Build history of the part. All positions in model axes, mm. Give positions to 0.01 mm unless a question says otherwise; leave off trailing zeros. Write each loop counter-clockwise with the first axis right and the second up, starting at its lowest first coordinate (ties: lowest second). Pieces come first, ordered by that corner, then holes. Notation, with made-up numbers: (60, 45) -> (70, 45) arc R28 ccw to (70, 70) -> close; hole circle Ø9 at (12.25, 36.25). An arc over 180 degrees is marked (long way). Write item = value, one per line. Start each with the question number.
Q1. Wall check: line 1 (Y direction, x = 50.8, z = 83.95); line 2 (X direction, y = 101.5, z = 83.9); line 3 (Y direction, x = 75.5, z = 84.2). Give the ranges that are in metal, low to high.
Q2. Mould opens along X. For faces 1 (the face through (88, 116, 85.725)), 2 (the face through (50.068, 198.315, 84.115)) say: pulls with the +X half, pulls with the -X half, needs draft (parallel to the pull), parting line crosses it, or undercut.
Q3. Drop a flat-ended pin along its axis: P1, Ø4, axis at x = 26.99, y = 127, coming from the -Z side (3 decimals). Give the stop position or say it passes through.
Q4. Saw through at B-B, the plane y = 177.8. List the corners of the cut face in (x, z) (3 decimals).
Q5. Saw through at A-A, the plane x = 127. List the corners of the cut face in (y, z) (3 decimals), then the cut area to 3 significant figures.
from build123d import *

# Parameters (mm, degrees)
F0_W      = 50.8
F0_H      = 177.8
F1_DEPTH  = 3.175
F3_DEPTH  = 76.2
F5_DEPTH  = 3.175
F7_D      = 6.7564
F7_DEPTH  = 29.21
F7_TIP    = 2.0298273432
F8_W      = 127
F8_H      = 177.8
F8_R      = 3.3782
F9_DEPTH  = 3.175
F10_W     = 247.0957003534
F10_H     = 423.9609837532
F11_DEPTH = 82.55


# Not quite as in the source:
# - an extrude ends at something that could not be found from the text; its depth is read off the source's solid


with BuildPart() as f1:
    # F0 (on Top) → F1 (new body)
    with BuildSketch(Plane.XY):
        Polygon((0, 228.6), (0, 177.8), (50.8, 177.8), (177.8, 177.8), (177.8, 228.6), align=None)
        with Locations((25.4, 88.9)):
            Rectangle(F0_W, F0_H)
    extrude(amount=F1_DEPTH)

    # F2 (on face) → F3 (join)
    with BuildSketch(Plane.XY.offset(3.175)):
        Polygon((3.175, 0), (3.175, 225.425), (177.8, 225.425), (177.8, 228.6), (0, 228.6), (0, 0), align=None)
    extrude(amount=F3_DEPTH)

    # F4 (on face) → F5 (join)
    with BuildSketch(Plane.XY.offset(79.375)):
        Polygon((177.8, 228.6), (0, 228.6), (0, 0), (3.175, 0), (3.175, 225.425), (177.8, 225.425), align=None)
        Polygon((177.8, 177.8), (177.8, 225.425), (3.175, 225.425), (3.175, 0), (50.8, 0), (50.8, 177.8), align=None)
    extrude(amount=F5_DEPTH)

    # F7
    with Locations(Plane.XY.offset(82.55)):
        with Locations((26.9875, 25.4), (26.9875, 50.8), (26.9875, 76.2), (26.9875, 101.6), (26.9875, 127), (26.9875, 152.4), (26.9875, 177.8), (50.8, 201.6125), (76.2, 201.6125), (101.6, 201.6125), (127, 201.6125), (152.4, 201.6125)):
            Hole(F7_D / 2, depth=F7_DEPTH)
            with Locations((0, 0, -(F7_DEPTH + F7_TIP / 2))):  # 118° drill point
                Cone(0, F7_D / 2, F7_TIP, mode=Mode.SUBTRACT)

    # F8 (on face) → F9 (join)
    with BuildSketch(Plane.XY.offset(82.55)):
        with Locations((114.3, 88.9)):
            Rectangle(F8_W, F8_H)
        Polygon((0, 228.6), (0, 0), (50.8, 0), (50.8, 177.8), (177.8, 177.8), (177.8, 228.6), align=None)
        with Locations((26.9875, 25.4)):
            Circle(F8_R, mode=Mode.SUBTRACT)
        with Locations((26.9875, 50.8)):
            Circle(F8_R, mode=Mode.SUBTRACT)
        with Locations((26.9875, 76.2)):
            Circle(F8_R, mode=Mode.SUBTRACT)
        with Locations((26.9875, 101.6)):
            Circle(F8_R, mode=Mode.SUBTRACT)
        with Locations((26.9875, 127)):
            Circle(F8_R, mode=Mode.SUBTRACT)
        with Locations((26.9875, 152.4)):
            Circle(F8_R, mode=Mode.SUBTRACT)
        with Locations((26.9875, 177.8)):
            Circle(F8_R, mode=Mode.SUBTRACT)
        with Locations((50.8, 201.6125)):
            Circle(F8_R, mode=Mode.SUBTRACT)
        with Locations((76.2, 201.6125)):
            Circle(F8_R, mode=Mode.SUBTRACT)
        with Locations((101.6, 201.6125)):
            Circle(F8_R, mode=Mode.SUBTRACT)
        with Locations((127, 201.6125)):
            Circle(F8_R, mode=Mode.SUBTRACT)
        with Locations((152.4, 201.6125)):
            Circle(F8_R, mode=Mode.SUBTRACT)
    extrude(amount=F9_DEPTH)

    # F10 (on Top) → F11 (cut, through all)
    with BuildSketch(Plane.XY):
        with Locations((80.0526309758, 75.9060680866)):
            Rectangle(F10_W, F10_H)
    extrude(amount=F11_DEPTH, mode=Mode.SUBTRACT)


solid = f1.part
Report:
q1.line_1 = 0 to 198.23, 204.99 to 228.6
q1.line_2 = 0 to 23.61, 30.36 to 177.8
q1.line_3 = 0 to 198.31, 204.92 to 228.6
q2.face_1 = needs draft
q2.face_2 = undercut
q3.P1 = through
q4.outline = (0, 82.55) -> (23.609, 82.55) -> (23.609, 85.725) -> (0, 85.725) -> close; (30.366, 82.55) -> (177.8, 82.55) -> (177.8, 85.725) -> (30.366, 85.725) -> close
q5.outline = (0, 82.55) -> (198.234, 82.55) -> (198.234, 85.725) -> (0, 85.725) -> close; (204.991, 82.55) -> (228.6, 82.55) -> (228.6, 85.725) -> (204.991, 85.725) -> close
q5.area = 704 mm2
